Could you check a few things on this drawing? It's one solid part, dimensions in mm from its lowest x, y, z. A direction names the side the tool comes from. Round coordinates to 2 decimals unless told otherwise and drop trailing zeros. Write each loop counter-clockwise with the first axis right and the second up, starting at its lowest first coordinate (ties: lowest second). Pieces come first, ordered by that corner, then holes. Notation, with made-up numbers: M 16,-2 L 38,-2 A30 ccw 38,30 Z; hole C 28.5,79.5 d4. An arc over 180 degrees is marked long. One line per item, written item: value. Start each with the question number.
(1) Which directions (+Z, -Z, +X, -X, +Y, -Y) give clear straight access to the entire face, cutting with the end or side of a thin tool? Please do the marked faces 1 and 2.
(2) I'm going to push flat-ended pins straight in: pin 1 Ø4 at (x, y) = (4.5, 31) entering from +Z; pin 2 Ø4 at (x, z) = (7, 5.5) entering from -Y; pin 3 Ø2 at (x, y) = (6.5, 14.5) entering from +Z; pin 4 Ø3 at (x, y) = (1, 34) entering from -Z. Where does each tip first touch, or does it pass through?
(3) I want a section at B-B on y = 24. Please give me the cut outline in (x, z).
(4) I want a section at A-A on x = 4. Please give me the cut outline in (y, z).
(5) If I drill on L1, parallel to Z at x = 6, y = 38; L2, parallel to X at y = 36, z = 3.5, over which ranges is the centre line in solid material (lowest first)?
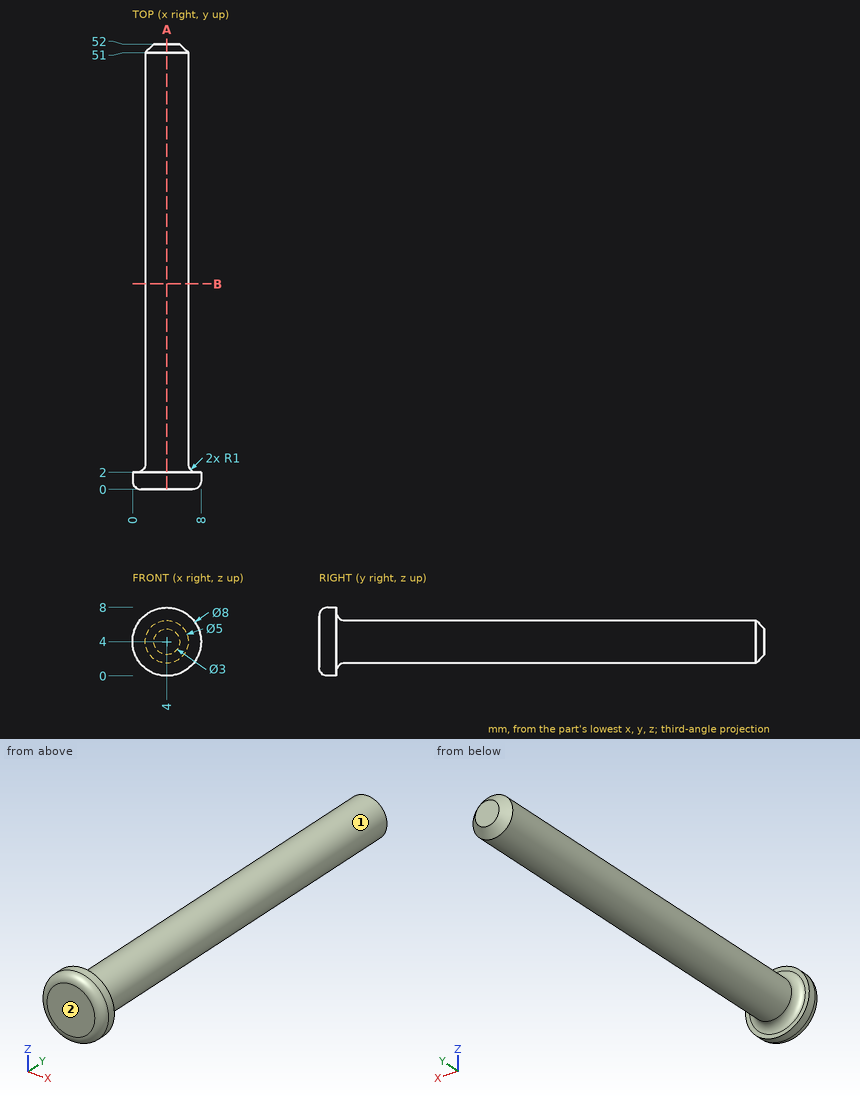
Found:
1. face 1: +Y
1. face 2: +Z, -Z, +X, -X, -Y
2. pin 1: stops at z = 6.5
2. pin 2: stops at y = 0
2. pin 3: stops at z = 6
2. pin 4: stops at z = 2
3. outline: C 4,4 d5
4. outline: M 0,1 A1 ccw 1,0 L 2,0 L 2,0.5 A1 cw 3,1.5 L 51,1.5 L 52,2.5 L 52,5.5 L 51,6.5 L 3,6.5 A1 cw 2,7.5 L 2,8 L 1,8 A1 ccw 0,7 Z
5. L1: z = 2.5 to 5.5
5. L2: x = 1.55 to 6.45
